Here's how the part is built. I have some questions about the finished solid (model axes, mm). Round coordinates to 2 decimals unless told otherwise and drop trailing zeros. Write each loop counter-clockwise with the first axis right and the second up, starting at its lowest first coordinate (ties: lowest second). Pieces come first, ordered by that corner, then holes. Notation, with made-up numbers: (-9.75, -32.75) -> (28.25, -32.75) arc R14 ccw to (28.25, -6.75) -> close; hole circle Ø9 at (87, -27.75). An arc over 180 degrees is marked (long way). Put each result on its own line as item: value. Start each with the question number.
1) I want a section at D-D, the plane x = -21. List the corners of the cut face in (y, z) for me, then the cut area to 3 significant figures.
2) I want a section at C-C, the plane y = -36. List the corners of the cut face in (x, z) for me, then the cut area to 3 significant figures.
3) I want a section at A-A, the plane z = 1.55. List the corners of the cut face in (x, y) for me.
4) Will these pins go through, and if not, where does the flat tip stop? P1, Ø1.1, axis at y = 8.5, z = 1.5, coming from the +X side; P2, Ø1.5, axis at x = -11.5, z = 1, coming from the -Y side (3 decimals); P3, Ø0.9, axis at x = -6, z = 1.5, coming from the -Y side.
5) If I drill on line 1 along Y through (x, z) = (42, 2.1); line 2 along X through (y, z) = (12.5, 1); line 3 along X through (y, z) = (13, 0.75), over which ranges is the centre line in solid material (lowest first)? Write a range as [from, to].
6) I want a section at B-B, the plane x = -11. List the corners of the cut face in (y, z) for me, then the cut area to 3 significant figures.
from build123d import *

# Parameters (mm, degrees)
SALIENTE_EXTRUIR1_DEPTH = 3
CORTAR_EXTRUIR1_REACH   = 71.508
CROQUIS4_W              = 3
CROQUIS4_H              = 1.42248357


with BuildPart() as part:
    # Croquis1 → Saliente-Extruir1 (new body)
    with BuildSketch(Plane.XY):
        with BuildLine():
            ThreePointArc((-31.713020554, -14.808252002), (-24.748737342, -24.748737342), (-14.808252002, -31.713020554))
            ThreePointArc((-14.808252002, -31.713020554), (0, -49.10376785), (14.808252002, -31.713020554))
            ThreePointArc((14.808252002, -31.713020554), (24.748737342, -24.748737342), (31.713020554, -14.808252002))
            ThreePointArc((31.713020554, -14.808252002), (49.10376785, 0), (31.713020554, 14.808252002))
            ThreePointArc((31.713020554, 14.808252002), (24.748737342, 24.748737342), (14.808252002, 31.713020554))
            ThreePointArc((14.808252002, 31.713020554), (0, 49.10376785), (-14.808252002, 31.713020554))
            ThreePointArc((-14.808252002, 31.713020554), (-24.748737342, 24.748737342), (-31.713020554, 14.808252002))
            ThreePointArc((-31.713020554, 14.808252002), (-49.10376785, 0), (-31.713020554, -14.808252002))
        make_face()
    extrude(amount=SALIENTE_EXTRUIR1_DEPTH)

    # Croquis4 → Cortar-Extruir1 (cut, up to next)
    with BuildSketch(Plane.XY.offset(3), mode=Mode.PRIVATE) as cortar_extruir1_sk1:
        with Locations((-5.30376785, -8.49072148)):
            Rectangle(CROQUIS4_W, CROQUIS4_H)
    cortar_extruir1_tool1 = extrude(cortar_extruir1_sk1.sketch, amount=-CORTAR_EXTRUIR1_REACH, mode=Mode.PRIVATE) & part.part
    # Croquis4 → Cortar-Extruir1 (cut, up to next)
    with BuildSketch(Plane.XY.offset(3), mode=Mode.PRIVATE) as cortar_extruir1_sk2:
        with Locations((-5.30376785, 8.49072148)):
            Rectangle(CROQUIS4_W, CROQUIS4_H)
    cortar_extruir1_tool2 = extrude(cortar_extruir1_sk2.sketch, amount=-CORTAR_EXTRUIR1_REACH, mode=Mode.PRIVATE) & part.part
    # Croquis4 → Cortar-Extruir1 (cut, up to next)
    with BuildSketch(Plane.XY.offset(3), mode=Mode.PRIVATE) as cortar_extruir1_sk3:
        with Locations((-11.10376785, 8.49072148)):
            Rectangle(CROQUIS4_W, CROQUIS4_H)
    cortar_extruir1_tool3 = extrude(cortar_extruir1_sk3.sketch, amount=-CORTAR_EXTRUIR1_REACH, mode=Mode.PRIVATE) & part.part
    # Croquis4 → Cortar-Extruir1 (cut, up to next)
    with BuildSketch(Plane.XY.offset(3), mode=Mode.PRIVATE) as cortar_extruir1_sk4:
        with Locations((-11.10376785, -8.49072148)):
            Rectangle(CROQUIS4_W, CROQUIS4_H)
    cortar_extruir1_tool4 = extrude(cortar_extruir1_sk4.sketch, amount=-CORTAR_EXTRUIR1_REACH, mode=Mode.PRIVATE) & part.part
    add(cortar_extruir1_tool1.solids().sort_by_distance((-5.303768, -8.490721, 3))[0], mode=Mode.SUBTRACT)
    add(cortar_extruir1_tool2.solids().sort_by_distance((-5.303768, 8.490721, 3))[0], mode=Mode.SUBTRACT)
    add(cortar_extruir1_tool3.solids().sort_by_distance((-11.103768, 8.490721, 3))[0], mode=Mode.SUBTRACT)
    add(cortar_extruir1_tool4.solids().sort_by_distance((-11.103768, -8.490721, 3))[0], mode=Mode.SUBTRACT)


solid = part.part
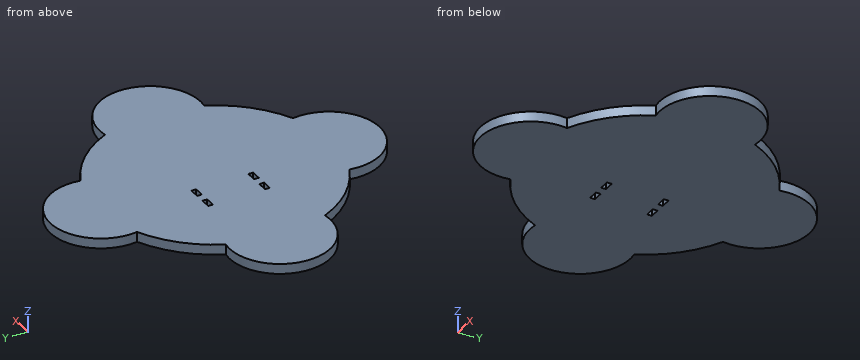
Findings:
1. outline: (-28, 0) -> (28, 0) -> (28, 3) -> (-28, 3) -> close
1. area: 168 mm2
2. outline: (-14.88, 0) -> (14.88, 0) -> (14.88, 3) -> (-14.88, 3) -> close
2. area: 89.3 mm2
3. outline: (-31.71, -14.81) arc R35 ccw to (-14.81, -31.71) arc R15 ccw (long way) to (14.81, -31.71) arc R35 ccw to (31.71, -14.81) arc R15 ccw (long way) to (31.71, 14.81) arc R35 ccw to (14.81, 31.71) arc R15 ccw (long way) to (-14.81, 31.71) arc R35 ccw to (-31.71, 14.81) arc R15 ccw (long way) to start; hole (-12.6, -9.2) -> (-9.6, -9.2) -> (-9.6, -7.78) -> (-12.6, -7.78) -> close; hole (-12.6, 7.78) -> (-9.6, 7.78) -> (-9.6, 9.2) -> (-12.6, 9.2) -> close; hole (-6.8, -9.2) -> (-3.8, -9.2) -> (-3.8, -7.78) -> (-6.8, -7.78) -> close; hole (-6.8, 7.78) -> (-3.8, 7.78) -> (-3.8, 9.2) -> (-6.8, 9.2) -> close
4. P1: stops at x = 46.82
4. P2: stops at y = -44.565
4. P3: stops at y = -48.04
5. line 1: y = [-12.75, 12.75]
5. line 2: x = [-42.4, 42.4]
5. line 3: x = [-41.59, 41.59]
6. outline: (-44.3, 0) -> (-9.2, 0) -> (-9.2, 3) -> (-44.3, 3) -> close; (-7.78, 0) -> (7.78, 0) -> (7.78, 3) -> (-7.78, 3) -> close; (9.2, 0) -> (44.3, 0) -> (44.3, 3) -> (9.2, 3) -> close
6. area: 257 mm2
